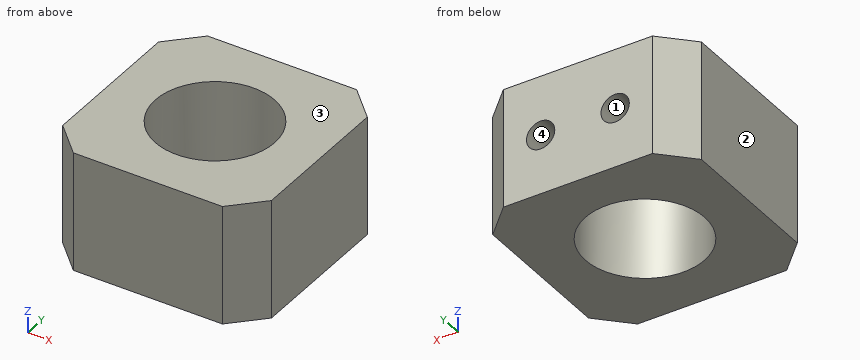
from build123d import *

# Parameters (mm, degrees)
SCHIZZO1_W                       = 7
SCHIZZO1_H                       = 7
SCHIZZO1_R                       = 2
ESTRUSIONE_ESTRUSIONE1_DEPTH     = 4
SMUSSO1_SIZE                     = 1
FORO_FILETTATO_M1_2X0_25_1_D     = 0.95
FORO_FILETTATO_M1_2X0_25_1_DEPTH = 1.2
FORO_FILETTATO_M1_2X0_25_1_TIP   = 0.285408794


with BuildPart() as part:
    # Schizzo1 → Estrusione-Estrusione1 (new body)
    with BuildSketch(Plane.XY):
        Rectangle(SCHIZZO1_W, SCHIZZO1_H)
        Circle(SCHIZZO1_R, mode=Mode.SUBTRACT)
    extrude(amount=ESTRUSIONE_ESTRUSIONE1_DEPTH)

    # Smusso1
    smusso1_edges = [part.edges().sort_by_distance(p)[0] for p in [
        (-3.5, 3.5, 2),
        (3.5, 3.5, 2),
        (3.5, -3.5, 2),
        (-3.5, -3.5, 2),
    ]]
    chamfer(smusso1_edges, length=SMUSSO1_SIZE)

    # Foro filettato M1.2x0.25-1
    with Locations(Plane(origin=(-1.25, 3.5, 2), x_dir=(1, 0, 0), z_dir=(0, 1, 0))):
        with Locations((0, 0), (2.5, 0)):
            Hole(FORO_FILETTATO_M1_2X0_25_1_D / 2, depth=FORO_FILETTATO_M1_2X0_25_1_DEPTH)
            with Locations((0, 0, -(FORO_FILETTATO_M1_2X0_25_1_DEPTH + FORO_FILETTATO_M1_2X0_25_1_TIP / 2))):  # 118° drill point
                Cone(0, FORO_FILETTATO_M1_2X0_25_1_D / 2, FORO_FILETTATO_M1_2X0_25_1_TIP, mode=Mode.SUBTRACT)


solid = part.part
The listing builds one solid part. Answer for the finished solid, in the listing's coordinates (mm). Face numbers are marked on the shaded views. Round coordinates to 2 decimals unless told otherwise and drop trailing zeros. Write each loop counter-clockwise with the first axis right and the second up, starting at its lowest first coordinate (ties: lowest second). Pieces come first, ordered by that corner, then holes. Notation, with made-up numbers: (27, 42) - (80, 42) arc R35 cw to (80, 80) - close; hole circle Ø3 at (53.5, 15). An arc over 180 degrees is marked (long way). Use a Markdown table: item, result. Add a question column.
1. The part is cut by section A-A (y = 0). Write down the section's boundary in (x, z), and give its area (3 significant figures).
2. For a pull along Z with two mould halves and no side action, classify the marked faces 1, 2, 3 and 4 as +Z half, -Z half, draft (parallel to the pull), parting line (faces both ways), or undercut.
3. The part is cut by section C-C (x = 0.25). Write down the section's boundary in (y, z), and give its area (3 significant figures).
4. Consider line 1 (X direction, y = 2.75, z = 2) (3 decimals); line 2 (Y direction, x = 0, z = 0.9); line 3 (Z direction, x = 1.25, y = 2.85) (3 decimals). Determine where each line is inside the solid, lowest interval first.
5. The part is cut by section B-B (z = 3.3). Write down the section's boundary in (x, y), and give its area (3 significant figures).
Reported:
| question | item | result |
|---|---|---|
| 1 | outline | (-3.5, 0) - (-2, 0) - (-2, 4) - (-3.5, 4) - close; (2, 0) - (3.5, 0) - (3.5, 4) - (2, 4) - close |
| 1 | area | 12.0 mm^2 |
| 2 | face 1 | undercut |
| 2 | face 2 | draft |
| 2 | face 3 | +Z half |
| 2 | face 4 | undercut |
| 3 | outline | (-3.5, 0) - (-1.98, 0) - (-1.98, 4) - (-3.5, 4) - close; (1.98, 0) - (3.5, 0) - (3.5, 4) - (1.98, 4) - close |
| 3 | area | 12.1 mm^2 |
| 4 | line 1 | -3.25 to -1.725, -0.775 to 0.775, 1.725 to 3.25 |
| 4 | line 2 | -3.5 to -2, 2 to 3.5 |
| 4 | line 3 | 0 to 1.525, 2.475 to 4 |
| 5 | outline | (-3.5, -2.5) - (-2.5, -3.5) - (2.5, -3.5) - (3.5, -2.5) - (3.5, 2.5) - (2.5, 3.5) - (-2.5, 3.5) - (-3.5, 2.5) - close; hole circle Ø4 at (0, 0) |
| 5 | area | 34.4 mm^2 |
